```python
from build123d import *

# Parameters (mm, degrees)
SKIZZE1_W                            = 152
SKIZZE1_H                            = 126
BASIS_BLECH1_DEPTH                   = 1.5
SKIZZIERTE_BIEGUNG2_DEPTH            = 152
SKIZZIERTE_BIEGUNG2_2_DEPTH          = 152
SKIZZIERTE_BIEGUNG3_DEPTH            = 152
SKIZZIERTE_BIEGUNG3_2_DEPTH          = 152
SKIZZIERTE_BIEGUNG4_DEPTH            = 152
SKIZZIERTE_BIEGUNG4_2_DEPTH          = 152
SCHNITT_LINEAR_AUSTRAGEN1_DEPTH      = 50
SCHNITT_LINEAR_AUSTRAGEN2_DEPTH      = 167.894252898
SCHNITT_LINEAR_AUSTRAGEN2_DEPTH_BACK = 167.894252898
SKIZZE15_W                           = 17
SKIZZE15_H                           = 4
SKIZZE22_R                           = 2.25
SCHNITT_LINEAR_AUSTRAGEN4_DEPTH      = 185.011324876
VERRUNDUNG3_R                        = 1
VERRUNDUNG4_R                        = 5
SCHNITT_LINEAR_AUSTRAGEN5_DEPTH      = 184.765876096


# Read off the part's stored shape, not the designer's step: Skizzierte Biegung2, Skizzierte Biegung3, Skizzierte Biegung4
# Sheet-metal steps are written as plain solids
with BuildPart() as part:
    # Skizze1 → Basis-Blech1 (new body)
    with BuildSketch(Plane.XY):
        with Locations((76, 63)):
            Rectangle(SKIZZE1_W, SKIZZE1_H)
    extrude(amount=-BASIS_BLECH1_DEPTH)

    # Skizzierte Biegung2 outline → Skizzierte Biegung2 (cut)
    with BuildSketch(Plane.YZ):
        with BuildLine():
            ThreePointArc((88.712436374, 0), (87.460340225, -1.102418411), (85.840155051, -1.5))
            Line((85.840155051, -1.5), (126, -1.5))
            Line((126, -1.5), (126, 0))
            Line((126, 0), (88.712436374, 0))
        make_face()
        with BuildLine():
            Line((0, -1.5), (40.159844949, -1.5))
            ThreePointArc((40.159844949, -1.5), (38.539659775, -1.102418411), (37.287563626, 0))
            Line((37.287563626, 0), (0, 0))
            Line((0, 0), (0, -1.5))
        make_face()
    extrude(amount=SKIZZIERTE_BIEGUNG2_DEPTH, mode=Mode.SUBTRACT)

    # Skizzierte Biegung2 2 outline → Skizzierte Biegung2 2 (add)
    with BuildSketch(Plane.YZ):
        with BuildLine():
            Line((85.840155051, 0), (88.712436374, 0))
            ThreePointArc((88.712436374, 0), (89.179540071, 0.951902827), (89.340155051, 2))
            Line((89.340155051, 2), (89.340155051, 37.840155051))
            Line((89.340155051, 37.840155051), (87.840155051, 37.840155051))
            Line((87.840155051, 37.840155051), (87.840155051, 2))
            ThreePointArc((87.840155051, 2), (87.254368613, 0.585786438), (85.840155051, 0))
        make_face()
        with BuildLine():
            ThreePointArc((36.659844949, 2), (36.820459929, 0.951902827), (37.287563626, 0))
            Line((37.287563626, 0), (40.159844949, 0))
            ThreePointArc((40.159844949, 0), (38.745631387, 0.585786438), (38.159844949, 2))
            Line((38.159844949, 2), (38.159844949, 37.840155051))
            Line((38.159844949, 37.840155051), (36.659844949, 37.840155051))
            Line((36.659844949, 37.840155051), (36.659844949, 2))
        make_face()
    extrude(amount=SKIZZIERTE_BIEGUNG2_2_DEPTH)

    # Skizzierte Biegung3 outline → Skizzierte Biegung3 (cut)
    with BuildSketch(Plane.YZ):
        with BuildLine():
            ThreePointArc((87.840155051, 25.840155051), (88.23773664, 27.460340225), (89.340155051, 28.712436374))
            Line((89.340155051, 28.712436374), (89.340155051, 37.840155051))
            Line((89.340155051, 37.840155051), (87.840155051, 37.840155051))
            Line((87.840155051, 37.840155051), (87.840155051, 25.840155051))
        make_face()
    extrude(amount=SKIZZIERTE_BIEGUNG3_DEPTH, mode=Mode.SUBTRACT)

    # Skizzierte Biegung3 2 outline → Skizzierte Biegung3 2 (add)
    with BuildSketch(Plane.YZ):
        with BuildLine():
            ThreePointArc((89.340155051, 25.840155051), (89.925941489, 27.254368613), (91.340155051, 27.840155051))
            Line((91.340155051, 27.840155051), (99.020465152, 27.840155051))
            Line((99.020465152, 27.840155051), (99.020465152, 29.340155051))
            Line((99.020465152, 29.340155051), (91.340155051, 29.340155051))
            ThreePointArc((91.340155051, 29.340155051), (90.292057878, 29.179540071), (89.340155051, 28.712436374))
            Line((89.340155051, 28.712436374), (89.340155051, 25.840155051))
        make_face()
    extrude(amount=SKIZZIERTE_BIEGUNG3_2_DEPTH)

    # Skizzierte Biegung4 outline → Skizzierte Biegung4 (cut)
    with BuildSketch(Plane.YZ):
        with BuildLine():
            Line((36.659844949, 37.840155051), (36.659844949, 28.712436374))
            ThreePointArc((36.659844949, 28.712436374), (37.76226336, 27.460340225), (38.159844949, 25.840155051))
            Line((38.159844949, 25.840155051), (38.159844949, 37.840155051))
            Line((38.159844949, 37.840155051), (36.659844949, 37.840155051))
        make_face()
    extrude(amount=SKIZZIERTE_BIEGUNG4_DEPTH, mode=Mode.SUBTRACT)

    # Skizzierte Biegung4 2 outline → Skizzierte Biegung4 2 (add)
    with BuildSketch(Plane.YZ):
        with BuildLine():
            Line((26.979534848, 29.340155051), (26.979534848, 27.840155051))
            Line((26.979534848, 27.840155051), (34.659844949, 27.840155051))
            ThreePointArc((34.659844949, 27.840155051), (36.074058511, 27.254368614), (36.659844949, 25.840155051))
            Line((36.659844949, 25.840155051), (36.659844949, 28.712436374))
            ThreePointArc((36.659844949, 28.712436374), (35.707942122, 29.179540071), (34.659844949, 29.340155051))
            Line((34.659844949, 29.340155051), (26.979534848, 29.340155051))
        make_face()
    extrude(amount=SKIZZIERTE_BIEGUNG4_2_DEPTH)

    # Skizze14 → Schnitt-Linear austragen1 (cut)
    with BuildSketch(Plane.ZY):
        with BuildLine():
            Line((29.340155051, 91.340155051), (29.340155051, 99.020465152))
            Line((29.340155051, 99.020465152), (27.840155051, 99.020465152))
            Line((27.840155051, 99.020465152), (27.840155051, 91.340155051))
            ThreePointArc((27.840155051, 91.340155051), (27.254368613, 89.925941488), (25.840155051, 89.340155051))
            Line((25.840155051, 89.340155051), (2, 89.340155051))
            ThreePointArc((2, 89.340155051), (-0.474873734, 88.315028785), (-1.5, 85.840155051))
            Line((-1.5, 85.840155051), (0, 85.840155051))
            ThreePointArc((0, 85.840155051), (0.585786438, 87.254368613), (2, 87.840155051))
            Line((2, 87.840155051), (25.840155051, 87.840155051))
            ThreePointArc((25.840155051, 87.840155051), (28.315028785, 88.865281317), (29.340155051, 91.340155051))
        make_face()
        with BuildLine():
            Line((0, 40.159844949), (-1.5, 40.159844949))
            ThreePointArc((-1.5, 40.159844949), (-0.474873734, 37.684971215), (2, 36.659844949))
            Line((2, 36.659844949), (25.840155051, 36.659844949))
            ThreePointArc((25.840155051, 36.659844949), (27.254368613, 36.074058512), (27.840155051, 34.659844949))
            Line((27.840155051, 34.659844949), (27.840155051, 26.979534848))
            Line((27.840155051, 26.979534848), (29.340155051, 26.979534848))
            Line((29.340155051, 26.979534848), (29.340155051, 34.659844949))
            ThreePointArc((29.340155051, 34.659844949), (28.315028785, 37.134718683), (25.840155051, 38.159844949))
            Line((25.840155051, 38.159844949), (2, 38.159844949))
            ThreePointArc((2, 38.159844949), (0.585786438, 38.745631387), (0, 40.159844949))
        make_face()
    schnitt_linear_austragen1 = extrude(amount=-SCHNITT_LINEAR_AUSTRAGEN1_DEPTH, mode=Mode.SUBTRACT)

    # Spiegeln1: Schnitt-Linear austragen1 across plane
    add(schnitt_linear_austragen1.mirror(Plane(origin=(76, 0, 0), x_dir=(0, 0, 1), z_dir=(1, 0, 0))), mode=Mode.SUBTRACT)

    # Skizze15 → Schnitt-Linear austragen2 (cut, two sides: drawn at the far end of the back side and taken through both)
    with BuildSketch(Plane.XZ.offset(-36.659844949).offset(-SCHNITT_LINEAR_AUSTRAGEN2_DEPTH_BACK)):
        with Locations((76, 15.5)):
            Rectangle(SKIZZE15_W, SKIZZE15_H)
    extrude(amount=SCHNITT_LINEAR_AUSTRAGEN2_DEPTH + SCHNITT_LINEAR_AUSTRAGEN2_DEPTH_BACK, mode=Mode.SUBTRACT)

    # Skizze22 → Schnitt-Linear austragen4 (cut, through all)
    with BuildSketch(Plane.XY.offset(29.340155051)):
        with Locations((63, 95.180310101)):
            Circle(SKIZZE22_R)
        with Locations((89, 95.180310101)):
            Circle(SKIZZE22_R)
        with Locations((63, 30.819689899)):
            Circle(SKIZZE22_R)
        with Locations((89, 30.819689899)):
            Circle(SKIZZE22_R)
    extrude(amount=-SCHNITT_LINEAR_AUSTRAGEN4_DEPTH, mode=Mode.SUBTRACT)

    # Verrundung3
    verrundung3_edges = [part.edges().sort_by_distance(p)[0] for p in [
        (67.5, 88.590155051, 13.5),
        (67.5, 37.409844949, 13.5),
        (67.5, 88.590155051, 17.5),
        (67.5, 37.409844949, 17.5),
        (84.5, 88.590155051, 17.5),
        (84.5, 37.409844949, 17.5),
        (84.5, 88.590155051, 13.5),
        (84.5, 37.409844949, 13.5),
    ]]
    fillet(verrundung3_edges, radius=VERRUNDUNG3_R)

    # Verrundung4
    verrundung4_edges = [part.edges().sort_by_distance(p)[0] for p in [
        (0, 85.840155051, -0.75),
        (152, 85.840155051, -0.75),
        (152, 40.159844949, -0.75),
        (0, 40.159844949, -0.75),
    ]]
    fillet(verrundung4_edges, radius=VERRUNDUNG4_R)

    # Skizze23 → Schnitt-Linear austragen5 (cut, through all)
    with BuildSketch(Plane.XY):
        with BuildLine():
            Line((3, 72), (5, 72))
            ThreePointArc((5, 72), (5.707106781, 71.707106781), (6, 71))
            Line((6, 71), (6, 55))
            ThreePointArc((6, 55), (5.707106781, 54.292893219), (5, 54))
            Line((5, 54), (3, 54))
            ThreePointArc((3, 54), (2.292893219, 54.292893219), (2, 55))
            Line((2, 55), (2, 71))
            ThreePointArc((2, 71), (2.292893219, 71.707106781), (3, 72))
        make_face()
        with BuildLine():
            Line((149, 72), (147, 72))
            ThreePointArc((147, 72), (146.292893219, 71.707106781), (146, 71))
            Line((146, 71), (146, 55))
            ThreePointArc((146, 55), (146.292893219, 54.292893219), (147, 54))
            Line((147, 54), (149, 54))
            ThreePointArc((149, 54), (149.707106781, 54.292893219), (150, 55))
            Line((150, 55), (150, 71))
            ThreePointArc((150, 71), (149.707106781, 71.707106781), (149, 72))
        make_face()
    extrude(amount=-SCHNITT_LINEAR_AUSTRAGEN5_DEPTH, mode=Mode.SUBTRACT)


solid = part.part
```
Here's how the part is built. I have some questions about the finished solid (model axes, mm). A direction names the side the tool comes from. Give positions to 0.01 mm unless a question says otherwise; leave off trailing zeros. Order: outer loops, then holes, each group sorted by start corner. A loop starts at its lowest first (then second) coordinate and runs counter-clockwise, first axis right, second up. Notation, with made-up numbers: M 40.5,50 L 77.5,50 A19 cw 77.5,57 Z; hole C 3.5,72 d11. An arc over 180 degrees is marked long. Use a Markdown table: item, result. Add a question column.
1. If we mould it in two halves opening along X, with no side actions, what happens to faces 1 (the flat face through (76, 31, 27.84)), 2 (the cylindrical face through (1.43, 84.34, -0.74)), 3 (the cylindrical face through (60.752, 30.919, 28.601))? For each: +X half, -X half, draft (parallel to the pull), parting line (faces both ways), or undercut.
2. I need wall thicknesses on probe 1 along Y at (x, z) = (63, 28.7); probe 2 along Y at (x, z) = (63, 28.5); probe 3 along Y at (x, z) = (83, 21.5). Which ranges of each line are inside material? Lowest first, please. Write a range as from..to.
3. Suppose I cut it at D-D (y = 43). List the corners of the cut face in (x, z) for me.
4. For pin 1 Ø23 at (x, y) = (93.5, 62) entering from +Z; pin 2 Ø3.5 at (x, y) = (89, 30.82) entering from +Z; pin 3 Ø12 at (x, z) = (64.5, 11) entering from +Y; pin 4 Ø1.7 at (y, z) = (38, 15.5) entering from -X, each with a flat end and sliding along its axis, tell me the tip position at first contact or that it passes through.
5. Suppose I cut it at C-C (x = 63.5). List the corners of the cut face in (y, z) for me, and give its area (3 significant figures).
6. Suppose I cut it at B-B (x = 89). List the corners of the cut face in (y, z) for me.
7. Suppose I cut it at A-A (z = 22.5). List the corners of the cut face in (x, y) for me.
8. On a 3-axis mill with a long thin cutter (end or side, diameter ignored), from which of +Z, -Z, +X, -X, +Y, -Y can I reach the whole of each face in a straight line? I mean faces 4 (the flat face through (76, 89.34, 11)), 5 (the flat face through (75, 63, 0)), 6 (the flat face through (76, 36.66, 11)). Say none if no direction works.
Results list:
| question | item | result |
|---|---|---|
| 1 | face 1 | draft |
| 1 | face 2 | -X half |
| 1 | face 3 | undercut |
| 2 | probe 1 | y = 26.98..28.57, 33.07..36.68, 89.32..92.93, 97.43..99.02 |
| 2 | probe 2 | y = 26.98..28.57, 33.07..36.93, 89.07..92.93, 97.43..99.02 |
| 2 | probe 3 | y = 36.66..38.16, 87.84..89.34 |
| 3 | outline | M 0.49,-1.5 L 151.51,-1.5 L 151.51,0 L 0.49,0 Z |
| 4 | pin 1 | stops at z = 0 |
| 4 | pin 2 | passes through |
| 4 | pin 3 | stops at y = 89.34 |
| 4 | pin 4 | stops at x = 50 |
| 5 | outline | M 26.98,27.84 L 28.63,27.84 L 28.63,29.34 L 26.98,29.34 Z; M 33.01,27.84 L 34.66,27.84 A2 cw 36.66,25.84 L 36.66,2 A3.5 ccw 40.16,-1.5 L 85.84,-1.5 A3.5 ccw 89.34,2 L 89.34,25.84 A2 cw 91.34,27.84 L 92.99,27.84 L 92.99,29.34 L 91.34,29.34 A3.5 ccw 87.84,25.84 L 87.84,2 A2 cw 85.84,0 L 40.16,0 A2 cw 38.16,2 L 38.16,25.84 A3.5 ccw 34.66,29.34 L 33.01,29.34 Z; M 97.37,27.84 L 99.02,27.84 L 99.02,29.34 L 97.37,29.34 Z |
| 5 | area | 176 mm² |
| 6 | outline | M 26.98,27.84 L 28.57,27.84 L 28.57,29.34 L 26.98,29.34 Z; M 33.07,27.84 L 34.66,27.84 A2 cw 36.66,25.84 L 36.66,2 A3.5 ccw 40.16,-1.5 L 85.84,-1.5 A3.5 ccw 89.34,2 L 89.34,25.84 A2 cw 91.34,27.84 L 92.93,27.84 L 92.93,29.34 L 91.34,29.34 A3.5 ccw 87.84,25.84 L 87.84,2 A2 cw 85.84,0 L 40.16,0 A2 cw 38.16,2 L 38.16,25.84 A3.5 ccw 34.66,29.34 L 33.07,29.34 Z; M 97.43,27.84 L 99.02,27.84 L 99.02,29.34 L 97.43,29.34 Z |
| 7 | outline | M 50,36.66 L 102,36.66 L 102,38.16 L 50,38.16 Z; M 50,87.84 L 102,87.84 L 102,89.34 L 50,89.34 Z |
| 8 | face 4 | -Z, +X, -X, +Y |
| 8 | face 5 | +Z, +X, -X |
| 8 | face 6 | -Z, +X, -X, -Y |
